from build123d import *

# Parameters (mm, degrees)
F1_DEPTH = 34.7990414
F2_R     = 3.69316
F3_R     = 1.98374
F4_R     = 2.032
F5_DEPTH = 26.1874
F6_R     = 2.82575


with BuildPart() as f1:
    # F0 (on Top) → F1 (new body)
    with BuildSketch(Plane.XY):
        Polygon((0, 7.63524), (0, 0), (-22.76856, 0), (-22.76856, 7.63524), (-24.47798, 7.63524), (-24.47798, -1.70942), (1.70942, -1.70942), (1.70942, 7.63524), align=None)
    extrude(amount=F1_DEPTH)

    # F2
    f2_edges = [f1.edges().sort_by_distance(p)[0] for p in [
        (1.70942, -1.70942, 17.399521),
        (-24.47798, -1.70942, 17.399521),
    ]]
    fillet(f2_edges, radius=F2_R)

    # F3
    f3_edges = [f1.edges().sort_by_distance(p)[0] for p in [
        (0, 0, 17.399521),
        (-22.76856, 0, 17.399521),
    ]]
    fillet(f3_edges, radius=F3_R)

    # F4 (on face) → F5 (cut, through all)
    with BuildSketch(Plane.YZ.offset(1.70942)):
        with Locations((4.80949, 2.82575)):
            Circle(F4_R)
        with Locations((4.80949, 31.9732914)):
            Circle(F4_R)
    extrude(amount=-F5_DEPTH, mode=Mode.SUBTRACT)

    # F6
    f6_edges = [f1.edges().sort_by_distance(p)[0] for p in [
        (0.85471, 7.63524, 34.799041),
        (-23.62327, 7.63524, 34.799041),
        (0.85471, 7.63524, 0),
        (-23.62327, 7.63524, 0),
    ]]
    fillet(f6_edges, radius=F6_R)


solid = f1.part
Geometry: final body of the model. Coordinates: model frame, mm. A direction names the side the tool comes from. Give positions to 0.01 mm unless a question says otherwise; leave off trailing zeros. Order: outer loops, then holes, each group sorted by start corner. A loop starts at its lowest first (then second) coordinate and runs counter-clockwise, first axis right, second up. Notation, with made-up numbers: (72, -24.5) -> (123, -24.5) arc R31 ccw to (123, 5.5) -> close; hole circle Ø8 at (61.5, -13.5). An arc over 180 degrees is marked (long way). Answer as a JSON object with one key per item and string values.
Q1. Material intervals for probe 1 along X at (y, z) = (4.25, 15.5); probe 2 along Y at (x, z) = (-8.5, 25); probe 3 along Z at (x, y) = (-23.25, 4.25), sorted ascending.
Entries:
{"probe 1": "x = -24.48 to -22.77, 0 to 1.71", "probe 2": "y = -1.71 to 0", "probe 3": "z = 0 to 0.87, 4.78 to 30.02, 33.93 to 34.8"}
Q2. Section D-D (z = 4). Output: boundary loops of the cut face in (x, y), plus the area to 3 significant figures.
Entries:
{"outline": "(-24.48, 1.98) arc R3.69 ccw to (-20.78, -1.71) -> (-1.98, -1.71) arc R3.69 ccw to (1.71, 1.98) -> (1.71, 3.15) -> (0, 3.15) -> (0, 1.98) arc R1.98 cw to (-1.98, 0) -> (-20.78, 0) arc R1.98 cw to (-22.77, 1.98) -> (-22.77, 3.15) -> (-24.48, 3.15) -> close; (-24.48, 6.47) -> (-22.77, 6.47) -> (-22.77, 7.64) -> (-24.48, 7.64) -> close; (0, 6.47) -> (1.71, 6.47) -> (1.71, 7.64) -> (0, 7.64) -> close", "area": "55.4 mm^2"}
Q3. First-contact query: pin 1 (2 mm diameter, centred on y = 0.5, z = 18.5, fed in from -X); pin 2 (2 mm diameter, centred on x = -16.5, z = 6, fed in from +Y). Flat tips, straight axial feed; report the tip coordinate or a pass-through.
Entries:
{"pin 1": "stops at x = -24.45", "pin 2": "stops at y = 0"}
Q4. Access query for faces 4 (the flat face through (-24, 7.635, 17)), 5 (the flat face through (0, 5, 17)). Directions: +Z, -Z, +X, -X, +Y, -Y. A direction counts if a zero-diameter tool reaches every point of the face in a straight line with its end or side. Return the directions, or none.
Entries:
{"face 4": "+Z, -Z, +X, -X, +Y", "face 5": "+Z, -Z, +Y"}
Q5. Section C-C (y = 1.5). Output: boundary loops of the cut face in (x, z).
Entries:
{"outline": "(-24.45, 0) -> (-22.71, 0) -> (-22.71, 34.8) -> (-24.45, 34.8) -> close; (-0.06, 0) -> (1.68, 0) -> (1.68, 34.8) -> (-0.06, 34.8) -> close"}
Q6. Draft query along X for faces 1 (the cylindrical face through (0.867, 6.748, 3.436)), 2 (the cylindrical face through (0.599, -0.656, 17.643)), 3 (the cylindrical face through (-22.203, 0.597, 17.643)). Return one class per face: released by +X, released by -X, zero draft, split by the parting line, or undercut.
Entries:
{"face 1": "zero draft", "face 2": "released by +X", "face 3": "undercut"}
Q7. Section A-A (y = 6). Output: boundary loops of the cut face in (x, z), plus the area to 3 significant figures.
Entries:
{"outline": "(-24.48, 0.26) -> (-22.77, 0.26) -> (-22.77, 1.18) -> (-24.48, 1.18) -> close; (-24.48, 4.47) -> (-22.77, 4.47) -> (-22.77, 30.33) -> (-24.48, 30.33) -> close; (-24.48, 33.62) -> (-22.77, 33.62) -> (-22.77, 34.54) -> (-24.48, 34.54) -> close; (0, 0.26) -> (1.71, 0.26) -> (1.71, 1.18) -> (0, 1.18) -> close; (0, 4.47) -> (1.71, 4.47) -> (1.71, 30.33) -> (0, 30.33) -> close; (0, 33.62) -> (1.71, 33.62) -> (1.71, 34.54) -> (0, 34.54) -> close", "area": "94.7 mm^2"}
Q8. Section B-B (z = 21). Output: boundary loops of the cut face in (x, y), plus the area to 3 significant figures.
Entries:
{"outline": "(-24.48, 1.98) arc R3.69 ccw to (-20.78, -1.71) -> (-1.98, -1.71) arc R3.69 ccw to (1.71, 1.98) -> (1.71, 7.64) -> (0, 7.64) -> (0, 1.98) arc R1.98 cw to (-1.98, 0) -> (-20.78, 0) arc R1.98 cw to (-22.77, 1.98) -> (-22.77, 7.64) -> (-24.48, 7.64) -> close", "area": "66.7 mm^2"}
